Autodesk Inventor part; units mm, degrees
ref_plane "YZ Plane" through (0, 0, 0) normal (1, 0, 0) x (0, 1, 0)
ref_plane "XZ Plane" through (0, 0, 0) normal (0, 1, 0) x (-1, 0, 0)
ref_plane "XY Plane" through (0, 0, 0) normal (0, 0, 1) x (1, 0, 0)
sketch "Sketch7" plane through (0, 0, 0) normal (0, 0, 1) x (1, 0, 0)
  line L0 (0, 0) -> (45, 0)
  line L1 (45, 0) -> (45, -63)
  line L2 (45, -63) -> (0, -63)
  line L3 (0, -63) -> (0, 0)
  dimension "d19" = 45
  dimension "d20" = 63
extrude "Extrusion3" add sketch "Sketch7" along normal blind 63
sketch "Sketch8" plane through (0, -63, 0) normal (0, -1, 0) x (1, 0, 0)
  line L0 (0, 0) -> (45, 0)
  line L1 (1.5, 0) -> (0, 0)
  line L2 (1.5, 1) -> (43.5, 1)
  line L3 (43.5, 1) -> (43.5, 61)
  line L4 (43.5, 61) -> (1.5, 61)
  line L5 (1.5, 61) -> (1.5, 1)
  dimension "d26" = 42
  dimension "d27" = 60
extrude "Extrusion4" cut sketch "Sketch8" against normal blind 63
sketch "Sketch9" plane through (0, 0, 63) normal (0, 0, 1) x (1, 0, 0)
  point P0 (0, 0)
sketch "Sketch10" plane through (0, -63, 0) normal (-1, 0, 0) x (0, 0, 1)
  line L0 (63, 0) -> (63, 63)
  line L1 (63, 0) -> (0, 0)
  line L2 (0, 0) -> (0, 6.1882)
  line L3 (0, 6.1882) -> (63, 6.1882)
  line L4 (63, 6.1882) -> (63, 0)
  point P0 (0, 63)
extrude "Extrusion5" add sketch "Sketch10" along normal blind 200
sketch "Sketch11" plane through (0, 0, 0) normal (-1, 0, 0) x (0, 0, 1)
  line L0 (63, -63) -> (63, 0)
  line L1 (0, 0) -> (0, -56.8118)
  line L2 (63, 0) -> (0, 0)
  line L3 (0, 0) -> (0, -56.8129)
  line L4 (0, -56.8129) -> (63, -56.8129)
  line L5 (63, -56.8129) -> (63, 0)
extrude "Extrusion6" add sketch "Sketch11" along normal blind 200
equation "\"BendRadius\" = Thickness"
equation "\"BendReliefWidth\" = Thickness"
equation "\"BendReliefDepth\" = 0.5 * Thickness"
equation "\"CornerReliefSize\" = 4 * Thickness"
equation "\"MinimumRemnant\" = 2 * Thickness"
equation "\"TransitionRadius\" = BendRadius"
equation "\"JacobiRadiusSize\" = BendRadius"
equation "\"GapSize\" = Thickness"
properties part number "soporte para motor"
Input: part model. Units: mm. Frame: model coordinates. A direction names the side the tool comes from. Give positions to 0.01 mm unless a question says otherwise; leave off trailing zeros. Order: outer loops, then holes, each group sorted by start corner. A loop starts at its lowest first (then second) coordinate and runs counter-clockwise, first axis right, second up. Notation, with made-up numbers: (83, 37) - (96, 37) arc R6 cw to (96, 41) - close; hole circle Ø5 at (-6, 40). An arc over 180 degrees is marked (long way). Use a Markdown table: item, result.
(1) Line query: line 1 (X direction, y = -6, z = 23); line 2 (Z direction, x = 4, y = -2.5). Output: solid intervals per line, ascending. Write a range as from..to.
Computed values:
| item | result |
|---|---|
| line 1 | x = -200..1.5, 43.5..45 |
| line 2 | z = 0..1, 61..63 |
(2) Draft query along X for faces 1 (the flat face through (22, -32, 1)), 2 (the flat face through (-200, -31, 31)), 3 (the flat face through (45, -31, 31)). Return one class per face: released by +X, released by -X, zero draft, split by the parting line, or undercut.
Computed values:
| item | result |
|---|---|
| face 1 | undercut |
| face 2 | released by -X |
| face 3 | released by +X |
(3) Section query A-A (x = 5). Output: boundary loops of the cut face in (y, z).
Computed values:
| item | result |
|---|---|
| outline | (-63, 0) - (0, 0) - (0, 1) - (-63, 1) - close; (-63, 61) - (0, 61) - (0, 63) - (-63, 63) - close |
(4) Section query B-B (z = 9.5). Output: boundary loops of the cut face in (x, y), then the cut area to 3 significant figures.
Computed values:
| item | result |
|---|---|
| outline | (-200, -63) - (1.5, -63) - (1.5, 0) - (-200, 0) - close; (43.5, -63) - (45, -63) - (45, 0) - (43.5, 0) - close |
| area | 12,800 mm2 |
(5) Access query for faces 4 (the flat face through (-76, -32, 0)), 5 (the flat face through (1.5, -32, 31)). Directions: +Z, -Z, +X, -X, +Y, -Y. A direction counts if a zero-diameter tool reaches every point of the face in a straight line with its end or side. Return the directions, or none.
Computed values:
| item | result |
|---|---|
| face 4 | -Z, +X, -X, +Y, -Y |
| face 5 | +Y, -Y |
(6) Section query C-C (y = -47). Output: boundary loops of the cut face in (x, z), then the cut area to 3 significant figures.
Computed values:
| item | result |
|---|---|
| outline | (-200, 0) - (45, 0) - (45, 63) - (-200, 63) - close; hole (1.5, 1) - (43.5, 1) - (43.5, 61) - (1.5, 61) - close |
| area | 12,900 mm2 |
